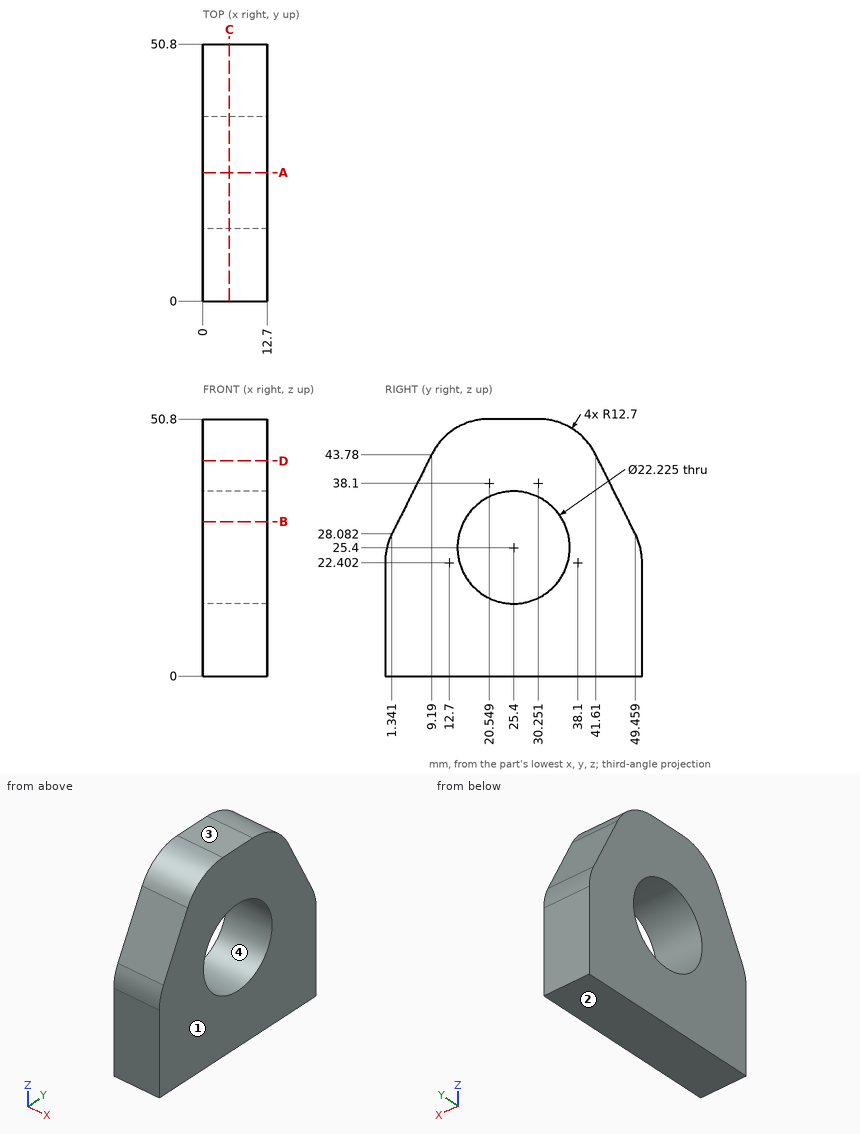
Verification items for this drawing (mm, ordinates from the low corner). Give positions to 0.01 mm unless a question says otherwise; leave off trailing zeros. Write each loop counter-clockwise with the first axis right and the second up, starting at its lowest first coordinate (ties: lowest second). Pieces come first, ordered by that corner, then holes. Notation, with made-up numbers: (50.5, 69) - (86.5, 69) arc R14 ccw to (86.5, 75) - close; hole circle Ø2 at (-31.5, 15.5). An arc over 180 degrees is marked (long way). Answer as a JSON object with one key per item and string values. Group by question number.
1) Release check for a two-part mould opening along Z. For the marked faces 1, 2, 3 and 4 record: pulls with the +Z half, pulls with the -Z half, needs draft (parallel to the pull), parting line crosses it, or undercut.
2) Sectioned sample at A-A (y = 25.4). Record the cut outline in (x, z).
3) Thickness scan on probe 1 along Z at (x, y) = (10.25, 25.4); probe 2 along Y at (x, z) = (6.5, 16.5) (1 decimal); probe 3 along Z at (x, y) = (8.5, 34) (1 decimal). Record the ranges inside material, lowest first. Write a range as from..to.
4) Sectioned sample at B-B (z = 30.5). Record the cut outline in (x, y), then the cut area to 3 significant figures.
5) Sectioned sample at C-C (x = 5.25). Record the cut outline in (y, z) (1 decimal), then the cut area to 3 significant figures.
6) Sectioned sample at D-D (z = 42.5). Record the cut outline in (x, y).
Geometry results:
{
 "1": {"face 1": "needs draft", "face 2": "pulls with the -Z half", "face 3": "pulls with the +Z half", "face 4": "undercut"},
 "2": {"outline": "(0, 0) - (12.7, 0) - (12.7, 14.29) - (0, 14.29) - close; (0, 36.51) - (12.7, 36.51) - (12.7, 50.8) - (0, 50.8) - close"},
 "3": {"probe 1": "z = 0..14.29, 36.51..50.8", "probe 2": "y = 0..18.7, 32.1..50.8", "probe 3": "z = 0..18.4, 32.4..50.2"},
 "4": {"outline": "(0, 2.55) - (12.7, 2.55) - (12.7, 15.53) - (0, 15.53) - close; (0, 35.27) - (12.7, 35.27) - (12.7, 48.25) - (0, 48.25) - close", "area": "330 mm^2"},
 "5": {"outline": "(0, 0) - (50.8, 0) - (50.8, 22.4) arc R12.7 ccw to (49.5, 28.1) - (41.6, 43.8) arc R12.7 ccw to (30.3, 50.8) - (20.5, 50.8) arc R12.7 ccw to (9.2, 43.8) - (1.3, 28.1) arc R12.7 ccw to (0, 22.4) - close; hole circle Ø22.2 at (25.4, 25.4)", "area": "1,850 mm^2"},
 "6": {"outline": "(0, 8.55) - (12.7, 8.55) - (12.7, 42.25) - (0, 42.25) - close"}
}
